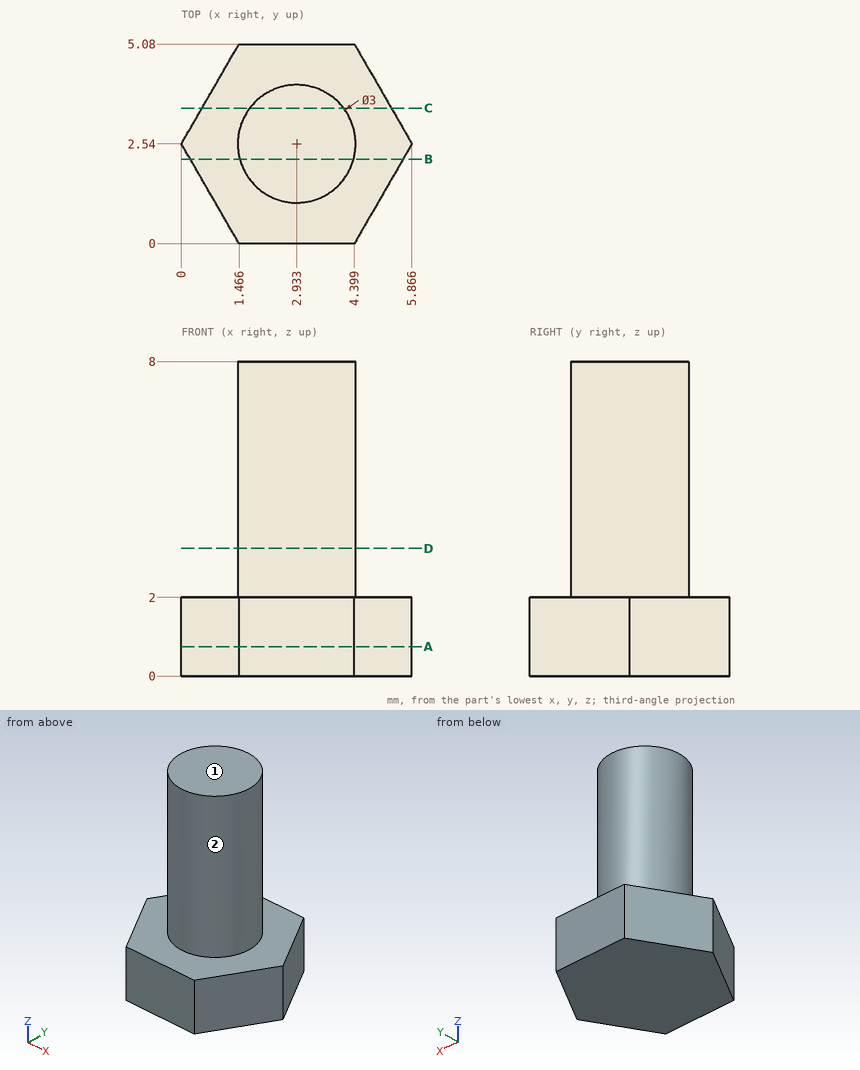
Verification items for this drawing (mm, ordinates from the low corner). A direction names the side the tool comes from. Give positions to 0.01 mm unless a question says otherwise; leave off trailing zeros. Write each loop counter-clockwise with the first axis right and the second up, starting at its lowest first coordinate (ties: lowest second). Pieces come first, ordered by that corner, then holes.
1) Section check C-C, the plane y = 3.45. Record the boundary of the cut face in (x, z) (1 decimal).
2) Material ranges on L1, parallel to Z at x = 3.35, y = 4.3; L2, parallel to Y at x = 2.9, z = 7.25; L3, parallel to X at y = 3.7, z = 0.5 (1 decimal), recorded low to high.
3) Access from +Z, -Z, +X, -X, +Y, -Y to the whole of each face (thin tool, end or side, straight path). Record for the marked faces 1 and 2.
4) Section check A-A, the plane z = 0.75. Record the boundary of the cut face in (x, y) (1 decimal).
5) Gauge pin test, flat end, axial feed: pin 1 (1.5 mm diameter, centred on y = 1.5, z = 1, fed in from +X). Record the tip position at first contact, or that the pin passes through.
6) Section check B-B, the plane y = 2.15. Record the boundary of the cut face in (x, z) (1 decimal).
7) Section check D-D, the plane z = 3.25. Record the boundary of the cut face in (x, y).
Computed:
1. outline: (0.5, 0) - (5.3, 0) - (5.3, 2) - (4.1, 2) - (4.1, 8) - (1.7, 8) - (1.7, 2) - (0.5, 2) - close
2. L1: z = 0 to 2
2. L2: y = 1.04 to 4.04
2. L3: x = 0.7 to 5.2
3. face 1: +Z, +X, -X, +Y, -Y
3. face 2: +Z
4. outline: (0, 2.5) - (1.5, 0) - (4.4, 0) - (5.9, 2.5) - (4.4, 5.1) - (1.5, 5.1) - close
5. pin 1: stops at x = 5.7
6. outline: (0.2, 0) - (5.6, 0) - (5.6, 2) - (4.4, 2) - (4.4, 8) - (1.5, 8) - (1.5, 2) - (0.2, 2) - close
7. outline: circle Ø3 at (2.93, 2.54)
